The listing builds one solid part. Answer for the finished solid, in the listing's coordinates (mm). Face numbers are marked on the shaded views. A direction names the side the tool comes from. Give positions to 0.01 mm unless a question says otherwise; leave off trailing zeros. Order: outer loops, then holes, each group sorted by start corner. A loop starts at its lowest first (then second) coordinate and runs counter-clockwise, first axis right, second up. Notation, with made-up numbers: (-31.75, -24.5) - (21.25, -24.5) arc R12 cw to (21.25, -8.5) - close; hole circle Ø10 at (-15.5, 36.25). An arc over 180 degrees is marked (long way). Write each question's results on one line, items separated by ' | '. Start each with the question number.
1. Flat-ended cylindrical pins translate along their axes: pin 1 (3 mm diameter, centred on y = 4, z = 29.5, fed in from -X); pin 2 (3 mm diameter, centred on x = 12.5, y = 3.5, fed in from -Z). Find the tip coordinate at first contact, or state that the pin passes through.
2. Determine the mould class of the marked faces 1, 2 and 3 for opening direction Z: released by +Z, released by -Z, zero draft, split by the parting line, or undercut.
3. Section C-C (y = 3) is taken. State how many separate pieces and enclosed holes the cut face has, and give its area (3 significant figures).
4. Section B-B (z = 11.5) is taken. Give the vertices of the cut face in (x, y), and give its area (3 significant figures).
5. Which of the six approach directions +Z, -Z, +X, -X, +Y, -Y give full straight-line access (tool end or side, diameter ignored) to the marked faces 4 and 5?
6. Find the intervals of material crossed by L1, parallel to X at y = 4.25, z = 0; L2, parallel to Z at x = -8.5, y = 3.5; L3, parallel to X at y = 2.5, z = -11, in increasing order.
7. Section A-A (z = 0) is taken. Give the vertices of the cut face in (x, y).
from build123d import *

# Parameters (mm, degrees)
SKETCH1_R           = 31.75
BOSS_EXTRUDE1_DEPTH = 6.35
CUT_EXTRUDE1_DEPTH  = 6.35
SKETCH3_R           = 1.500000048
SKETCH3_W           = 6.35
SKETCH3_H           = 6.35
CUT_EXTRUDE2_DEPTH  = 6.35
SKETCH4_R           = 1.016
CUT_EXTRUDE3_DEPTH  = 6.35


with BuildPart() as part:
    # Sketch1 → Boss-Extrude1 (new body)
    with BuildSketch(Plane(origin=(0, 0, 0), x_dir=(1, 0, 0), z_dir=(0, 1, 0))):
        with Locations(Location((0, 0, 0), (0, 0, 270))):
            Circle(SKETCH1_R)
    extrude(amount=BOSS_EXTRUDE1_DEPTH)

    # Sketch2 → Cut-Extrude1 (cut)
    with BuildSketch(Plane(origin=(0, 6.35, 0), x_dir=(1, 0, 0), z_dir=(0, 1, 0))):
        Polygon((3.782860755, 31.523839622), (3.026288604, 25.219071698), (0, 25.58222633), (0, 31.75), (0, 34.308222633), (4.087660755, 34.063839622), align=None)
        Polygon((14.336514482, 28.328904894), (11.469211586, 22.663123915), (8.749636716, 24.039429306), (10.859139551, 29.83524071), (11.734103222, 32.239183641), (15.491663957, 30.611476411), align=None)
        Polygon((23.160972979, 21.717086146), (18.528778383, 17.373668917), (16.443938113, 19.597122323), (20.408506608, 24.321911069), (22.052900419, 26.281623301), (25.027143854, 23.466917368), align=None)
        Polygon((29.191876315, 12.485866298), (23.353501052, 9.988693039), (22.154857887, 12.791113165), (27.49630657, 15.875), (29.711792359, 17.154111317), (31.54398084, 13.491901755), align=None)
        Polygon((31.701808541, 1.748666704), (25.361446833, 1.398933363), (25.193574829, 4.442306983), (31.267646158, 5.513329641), (33.787003641, 5.957560339), (34.256148198, 1.889563672), align=None)
        Polygon((30.388034788, -9.199447903), (24.31042783, -7.359558323), (25.193574829, -4.442306983), (31.267646158, -5.513329641), (33.787003641, -5.957560339), (32.836518516, -9.940683678), align=None)
        Polygon((25.40901556, -19.037973323), (20.327212448, -15.230378659), (22.154857887, -12.791113165), (27.49630657, -15.875), (29.711792359, -17.154111317), (27.456320086, -20.571937867), align=None)
        Polygon((17.365294059, -26.58023819), (13.892235247, -21.264190552), (16.443938113, -19.597122323), (20.408506608, -24.321911069), (22.052900419, -26.281623301), (18.764484241, -28.721912739), align=None)
        Polygon((7.227061809, -30.916534049), (5.781649447, -24.733227239), (8.749636716, -24.039429306), (10.859139551, -29.83524071), (11.734103222, -32.239183641), (7.809374662, -33.407601046), align=None)
        Polygon((-3.782860755, -31.523839622), (-3.026288604, -25.219071698), (0, -25.58222633), (0, -31.75), (0, -34.308222633), (-4.087660755, -34.063839622), align=None)
        Polygon((-14.336514482, -28.328904894), (-11.469211586, -22.663123915), (-8.749636716, -24.039429306), (-10.859139551, -29.83524071), (-11.734103222, -32.239183641), (-15.491663957, -30.611476411), align=None)
        Polygon((-23.160972979, -21.717086146), (-18.528778383, -17.373668917), (-16.443938113, -19.597122323), (-20.408506608, -24.321911069), (-22.052900419, -26.281623301), (-25.027143854, -23.466917368), align=None)
        Polygon((-29.191876315, -12.485866298), (-23.353501052, -9.988693039), (-22.154857887, -12.791113165), (-27.49630657, -15.875), (-29.711792359, -17.154111317), (-31.54398084, -13.491901755), align=None)
        Polygon((-31.701808541, -1.748666704), (-25.361446833, -1.398933363), (-25.193574829, -4.442306983), (-31.267646158, -5.513329641), (-33.787003641, -5.957560339), (-34.256148198, -1.889563672), align=None)
        Polygon((-30.388034788, 9.199447903), (-24.31042783, 7.359558323), (-25.193574829, 4.442306983), (-31.267646158, 5.513329641), (-33.787003641, 5.957560339), (-32.836518516, 9.940683678), align=None)
        Polygon((-25.40901556, 19.037973323), (-20.327212448, 15.230378659), (-22.154857887, 12.791113165), (-27.49630657, 15.875), (-29.711792359, 17.154111317), (-27.456320086, 20.571937867), align=None)
        Polygon((-17.365294059, 26.58023819), (-13.892235247, 21.264190552), (-16.443938113, 19.597122323), (-20.408506608, 24.321911069), (-22.052900419, 26.281623301), (-18.764484241, 28.721912739), align=None)
        Polygon((-7.227061809, 30.916534049), (-5.781649447, 24.733227239), (-8.749636716, 24.039429306), (-10.859139551, 29.83524071), (-11.734103222, 32.239183641), (-7.809374662, 33.407601046), align=None)
    extrude(amount=-CUT_EXTRUDE1_DEPTH, mode=Mode.SUBTRACT)

    # Sketch3 → Cut-Extrude2 (cut)
    with BuildSketch(Plane(origin=(0, 6.35, 0), x_dir=(1, 0, 0), z_dir=(0, 1, 0))):
        with Locations(Location((0, 0, 0), (0, 0, 270))):
            Circle(SKETCH3_R)
        Polygon((-2.330369343, -10.386318102), (-5.505369343, -15.885579416), (-11.004630657, -12.710579416), (-7.829630657, -7.211318102), align=None)
        Polygon((-7.829630657, 7.211318102), (-11.004630657, 12.710579416), (-5.505369343, 15.885579416), (-2.330369343, 10.386318102), align=None)
        with Locations((13.335, 0)):
            Rectangle(SKETCH3_W, SKETCH3_H)
    extrude(amount=-CUT_EXTRUDE2_DEPTH, mode=Mode.SUBTRACT)

    # Sketch4 → Cut-Extrude3 (cut)
    with BuildSketch(Plane(origin=(0, 6.35, 0), x_dir=(1, 0, 0), z_dir=(0, 1, 0))):
        with Locations(Location((6.35, 0, 0), (0, 0, 270))):
            Circle(SKETCH4_R)
        with Locations(Location((0, -6.35, 0), (0, 0, 270))):
            Circle(SKETCH4_R)
        with Locations(Location((-6.35, 0, 0), (0, 0, 270))):
            Circle(SKETCH4_R)
        with Locations(Location((0, 6.35, 0), (0, 0, 270))):
            Circle(SKETCH4_R)
    extrude(amount=-CUT_EXTRUDE3_DEPTH, mode=Mode.SUBTRACT)


solid = part.part
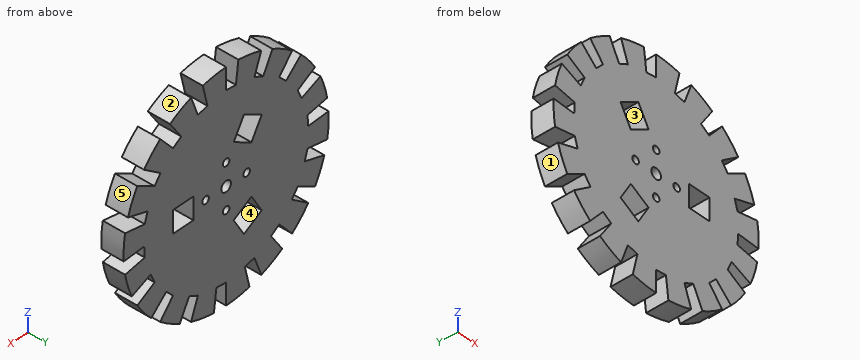
Reported:
1) pin 1: x = -14.97 | pin 2: z = -27.66
2) face 1: released by -Z | face 2: released by +Z | face 3: undercut
3) separate pieces: 1 | enclosed holes: 8 | area: 2,640 mm²
4) outline: (-29.59, 0) - (-26.89, 0) - (-26.89, 6.35) - (-29.59, 6.35) - close; (-22.71, 0) - (-10.31, 0) - (-10.31, 6.35) - (-22.71, 6.35) - close; (-2.97, 0) - (29.59, 0) - (29.59, 6.35) - (-2.97, 6.35) - close | area: 303 mm²
5) face 4: +Y, -Y | face 5: +Z, +X, +Y, -Y
6) L1: -31.75 to -7.37, -5.33 to -1.5, 1.5 to 5.33, 7.37 to 10.16, 16.51 to 31.75 | L2: -24.1 to -14.16, -8.37 to 8.37, 14.16 to 30.59 | L3: -29.78 to -10.02, -2.68 to 22.92, 25.72 to 29.78
7) outline: (-31.75, 0) - (-7.37, 0) - (-7.37, 6.35) - (-31.75, 6.35) - close; (-5.33, 0) - (-1.5, 0) - (-1.5, 6.35) - (-5.33, 6.35) - close; (1.5, 0) - (5.33, 0) - (5.33, 6.35) - (1.5, 6.35) - close; (7.37, 0) - (10.16, 0) - (10.16, 6.35) - (7.37, 6.35) - close; (16.51, 0) - (31.75, 0) - (31.75, 6.35) - (16.51, 6.35) - close
